Here's the drawing with two shaded views (mm, measured from the low corner). I have some questions. A direction names the side the tool comes from. Give positions to 0.01 mm unless a question says otherwise; leave off trailing zeros. Order: outer loops, then holes, each group sorted by start corner. A loop starts at its lowest first (then second) coordinate and runs counter-clockwise, first axis right, second up. Notation, with made-up numbers: M -21.75,79.5 L 22.25,79.5 A24 ccw 22.25,99.5 Z; hole C -14.5,64 d4. An arc over 180 degrees is marked long. Write each question's results on one line, items separated by ' | '.
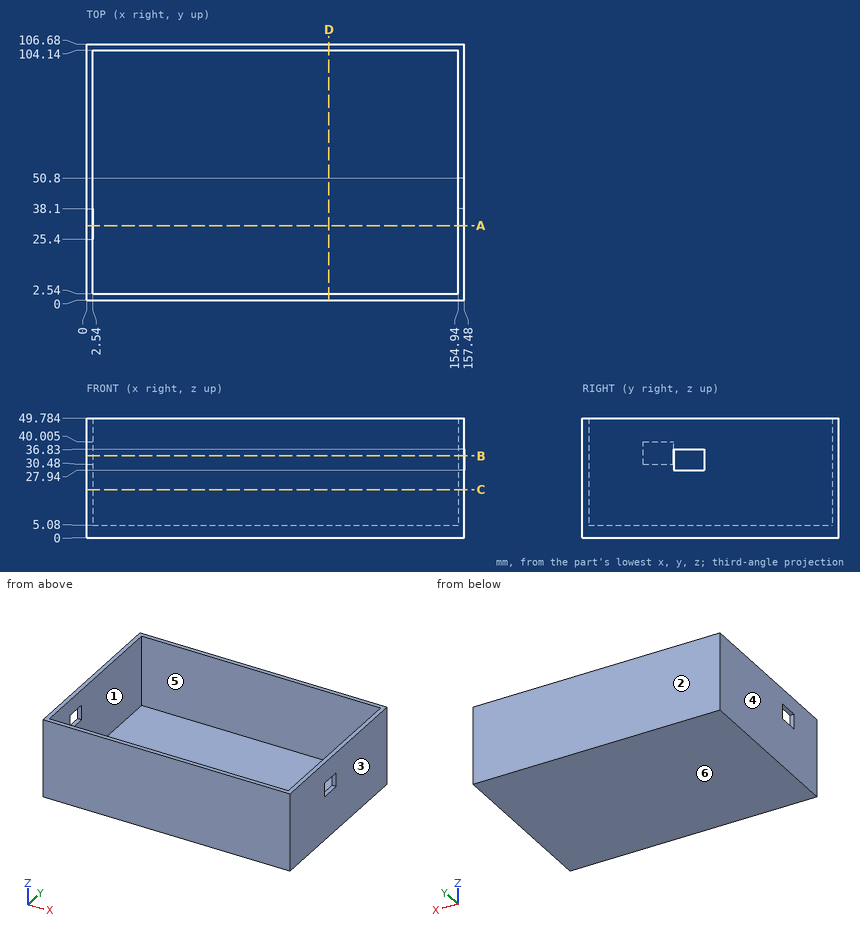
(1) Imagine slicing it at A-A, the plane y = 31. Write out the boundary of the cut face in (x, z) (3 decimals).
Data:
outline: M 0,0 L 157.48,0 L 157.48,49.784 L 154.94,49.784 L 154.94,5.08 L 2.54,5.08 L 2.54,30.48 L 0,30.48 Z; M 0,40.005 L 2.54,40.005 L 2.54,49.784 L 0,49.784 Z
(2) Imagine slicing it at D-D, the plane x = 101. Write out the boundary of the cut face in (y, z).
Data:
outline: M 0,0 L 106.68,0 L 106.68,49.78 L 104.14,49.78 L 104.14,5.08 L 2.54,5.08 L 2.54,49.78 L 0,49.78 Z
(3) Imagine slicing it at B-B, the plane z = 34. Write out the boundary of the cut face in (x, y), plus the area to 3 significant figures.
Data:
outline: M 0,0 L 157.48,0 L 157.48,38.1 L 154.94,38.1 L 154.94,2.54 L 2.54,2.54 L 2.54,25.4 L 0,25.4 Z; M 0,38.1 L 2.54,38.1 L 2.54,104.14 L 154.94,104.14 L 154.94,50.8 L 157.48,50.8 L 157.48,106.68 L 0,106.68 Z | area: 1,250 mm2
(4) Imagine slicing it at C-C, the plane z = 20. Write out the boundary of the cut face in (x, y), plus the area to 3 significant figures.
Data:
outline: M 0,0 L 157.48,0 L 157.48,106.68 L 0,106.68 Z; hole M 2.54,2.54 L 154.94,2.54 L 154.94,104.14 L 2.54,104.14 Z | area: 1,320 mm2
(5) For the marked faces 1 and 2, which set-ups out of +Z, -Z, +X, -X, +Y, -Y let a thin tool reach every point of the face, with its end or its side?
Data:
face 1: +Z | face 2: +Z, -Z, +X, -X, +Y
(6) I need wall thicknesses on L1, parallel to X at y = 51, z = 28.5; L2, parallel to Y at x = 93, z = 15; L3, parallel to Z at x = 100.5, y = 65. Which ranges of each line are inside material? Lowest first, please. Write a range as from..to.
Data:
L1: x = 0..2.54, 154.94..157.48 | L2: y = 0..2.54, 104.14..106.68 | L3: z = 0..5.08
(7) We'd pull the mould along X, two halves only. Please class the marked faces 3, 4, 5 and 6: +X half, -X half, draft (parallel to the pull), parting line (faces both ways), or undercut.
Data:
face 3: +X half | face 4: -X half | face 5: undercut | face 6: draft
(8) Will this pin go through, and if not, where does the flat tip stop? P1, Ø1, axis at x = 108.5, y = 19.5, coming from the +Z side.
Data:
P1: stops at z = 5.08
